Check sheet for the modelled part. Datum: model origin and axes. Units: mm. A direction names the side the tool comes from. Give positions to 0.01 mm unless a question says otherwise; leave off trailing zeros. Loops run counter-clockwise (first coordinate to the right, second up) from the corner with the lowest first, then second, coordinate; pieces in that order, holes last. Notation, with made-up numbers: (-10.5, -22.75) - (35.5, -22.75) arc R28 ccw to (35.5, -2.75) - close; hole circle Ø5 at (-16.75, 15.25). An arc over 180 degrees is marked (long way). Use CSV: the item, a comma, the result in double quotes.
from build123d import *

# Parameters (mm, degrees)
SKETCH1_W           = 15
SKETCH1_H           = 15
BOSS_EXTRUDE1_DEPTH = 20
CUT_EXTRUDE1_START  = -3
SKETCH2_W           = 12.5
SKETCH2_H           = 12.5
CUT_EXTRUDE1_DEPTH  = 17
BOSS_EXTRUDE3_DEPTH = 15
SKETCH6_R           = 1.5
CUT_EXTRUDE2_DEPTH  = 33.210246817
SKETCH7_R           = 1.5
CUT_EXTRUDE3_DEPTH  = 33.210246817


with BuildPart() as part:
    # Sketch1 → Boss-Extrude1 (new body)
    with BuildSketch(Plane(origin=(0, 0, 0), x_dir=(1, 0, 0), z_dir=(0, 1, 0))):
        Rectangle(SKETCH1_W, SKETCH1_H)
    extrude(amount=BOSS_EXTRUDE1_DEPTH)

    # Sketch2 → Cut-Extrude1 (cut)
    with BuildSketch(Plane(origin=(0, 20, 0), x_dir=(1, 0, 0), z_dir=(0, 1, 0)).offset(CUT_EXTRUDE1_START)):
        Rectangle(SKETCH2_W, SKETCH2_H)
    extrude(amount=-CUT_EXTRUDE1_DEPTH, mode=Mode.SUBTRACT)

    # Sketch5 → Boss-Extrude3 (add, through all)
    with BuildSketch(Plane(origin=(0, 0, -7.5), x_dir=(-1, 0, 0), z_dir=(0, 0, -1))):
        with BuildLine():
            Line((-7.5, 20), (7.5, 20))
            ThreePointArc((7.5, 20), (0, 27.5), (-7.5, 20))
        make_face()
    extrude(amount=-BOSS_EXTRUDE3_DEPTH)

    # Sketch6 → Cut-Extrude2 (cut, through all)
    with BuildSketch(Plane(origin=(7.5, 0, 0), x_dir=(0, 0, -1), z_dir=(1, 0, 0))):
        with Locations((0, 11.096857515)):
            Circle(SKETCH6_R)
    extrude(amount=-CUT_EXTRUDE2_DEPTH, mode=Mode.SUBTRACT)

    # Sketch7 → Cut-Extrude3 (cut, through all)
    with BuildSketch(Plane.XY.offset(7.5)):
        with Locations((0, 20)):
            Circle(SKETCH7_R)
    extrude(amount=-CUT_EXTRUDE3_DEPTH, mode=Mode.SUBTRACT)


solid = part.part
1. Sectioned sample at A-A, the plane z = 0. Record the boundary of the cut face in (x, y), and give its area (3 significant figures).
Completed:
outline,"(-7.5, 0) - (-6.25, 0) - (-6.25, 9.6) - (-7.5, 9.6) - close; (-7.5, 12.6) - (-6.25, 12.6) - (-6.25, 17) - (6.25, 17) - (6.25, 12.6) - (7.5, 12.6) - (7.5, 20) arc R7.5 ccw to (-7.5, 20) - close; (6.25, 0) - (7.5, 0) - (7.5, 9.6) - (6.25, 9.6) - close; hole circle Ø3 at (0, 20)"
area,"161 mm²"
2. Scan lines: line 1 along X through (y, z) = (4.25, 0); line 2 along Y through (x, z) = (0, -2.5). Record each from-to range of solid material in increasing order.
Completed:
line 1,"x = -7.5 to -6.25, 6.25 to 7.5"
line 2,"y = 17 to 18.5, 21.5 to 27.5"
3. Sectioned sample at C-C, the plane y = 3. Record the boundary of the cut face in (x, z).
Completed:
outline,"(-7.5, -7.5) - (7.5, -7.5) - (7.5, 7.5) - (-7.5, 7.5) - close; hole (-6.25, -6.25) - (6.25, -6.25) - (6.25, 6.25) - (-6.25, 6.25) - close"
4. Sectioned sample at D-D, the plane x = -4. Record the boundary of the cut face in (y, z).
Completed:
outline,"(0, -7.5) - (26.34, -7.5) - (26.34, 7.5) - (0, 7.5) - (0, 6.25) - (17, 6.25) - (17, -6.25) - (0, -6.25) - close"
5. Release check for a two-part mould opening along Z. For faces 1 (the face through (0, 14, -7.5)), 2 (the face through (0, 9, 6.25)), 3 (the face through (7.5, 10, 2)) record: released by +Z, released by -Z, zero draft, split by the parting line, or undercut.
Completed:
face 1,"released by -Z"
face 2,"undercut"
face 3,"zero draft"
6. Set-up check for faces 4 (the face through (0, 14, 7.5)), 5 (the face through (-6.25, 9, 0)): record each of +Z, -Z, +X, -X, +Y, -Y from which the full face is reachable in a straight line by a thin tool's end or side.
Completed:
face 4,"+Z, +X, -X, +Y, -Y"
face 5,"-Y"
7. Sectioned sample at B-B, the plane x = 0. Record the boundary of the cut face in (y, z).
Completed:
outline,"(0, -7.5) - (18.5, -7.5) - (18.5, 7.5) - (0, 7.5) - (0, 6.25) - (17, 6.25) - (17, -6.25) - (0, -6.25) - close; (21.5, -7.5) - (27.5, -7.5) - (27.5, 7.5) - (21.5, 7.5) - close"
8. Go/stop test with flat-tipped pins: pin 1 Ø4 at (x, z) = (3.5, -5) entering from +Y; pin 2 Ø4 at (x, z) = (0, 0) entering from -Y. Record where each tip stops, or that it passes through.
Completed:
pin 1,"stops at y = 27.35"
pin 2,"stops at y = 17"
